Part print with two shaded views. Sizes in mm from the minimum x, y, z corner. Give positions to 0.01 mm unless a question says otherwise; leave off trailing zeros. Loops run counter-clockwise (first coordinate to the right, second up) from the corner with the lowest first, then second, coordinate; pieces in that order, holes last. Notation, with made-up numbers: M 67,42.25 L 89,42.25 A27 ccw 89,75.25 Z; hole C 32,3 d4. An arc over 180 degrees is marked long. Answer in a Markdown table with one row per item.
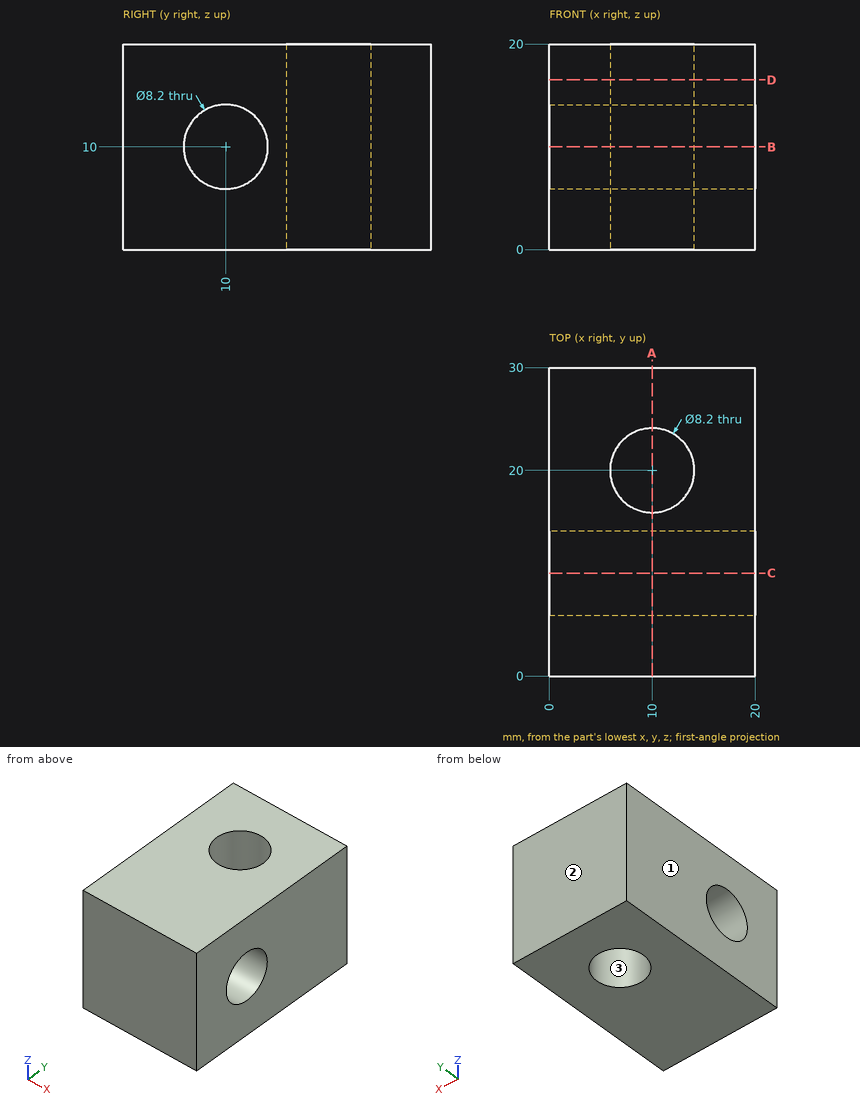
Q1. Saw through at B-B (z = 10). Give the cut face in (x, y).
Reported:
| item | result |
|---|---|
| outline | M 0,0 L 20,0 L 20,5.9 L 0,5.9 Z; M 0,14.1 L 20,14.1 L 20,30 L 0,30 Z; hole C 10,20 d8.2 |
Q2. Drop a flat-ended pin along its axis: pin 1 (3 mm diameter, centred on x = 9.5, y = 19, fed in from -Z). Give the stop position or say it passes through.
Reported:
| item | result |
|---|---|
| pin 1 | through |
Q3. Probe probe 1 along Z at (x, y) = (5.75, 10); probe 2 along Y at (x, z) = (12, 9); probe 3 along X at (y, z) = (18.25, 2). List the from-to ranges inside material, lowest first.
Reported:
| item | result |
|---|---|
| probe 1 | 0 to 5.9, 14.1 to 20 |
| probe 2 | 0 to 6.02, 13.98 to 16.42, 23.58 to 30 |
| probe 3 | 0 to 6.29, 13.71 to 20 |
Q4. Saw through at A-A (x = 10). Give the cut face in (y, z), and give its area (3 significant figures).
Reported:
| item | result |
|---|---|
| outline | M 0,0 L 15.9,0 L 15.9,20 L 0,20 Z; M 24.1,0 L 30,0 L 30,20 L 24.1,20 Z; hole C 10,10 d8.2 |
| area | 383 mm² |
Q5. Saw through at C-C (y = 10). Give the cut face in (x, z).
Reported:
| item | result |
|---|---|
| outline | M 0,0 L 20,0 L 20,5.9 L 0,5.9 Z; M 0,14.1 L 20,14.1 L 20,20 L 0,20 Z |
Q6. Saw through at D-D (z = 16.5). Give the cut face in (x, y).
Reported:
| item | result |
|---|---|
| outline | M 0,0 L 20,0 L 20,30 L 0,30 Z; hole C 10,20 d8.2 |
Q7. Mould opens along Y. For the marked faces 1, 2 and 3 say: released by +Y, released by -Y, zero draft, split by the parting line, or undercut.
Reported:
| item | result |
|---|---|
| face 1 | zero draft |
| face 2 | released by +Y |
| face 3 | undercut |
